Check sheet for the modelled part. Datum: model origin and axes. Units: mm. Face numbers are marked on the shaded views. A direction names the side the tool comes from. Round coordinates to 2 decimals unless told otherwise and drop trailing zeros. Order: outer loops, then holes, each group sorted by start corner. A loop starts at its lowest first (then second) coordinate and runs counter-clockwise, first axis right, second up.
Q1. Scan lines: probe 1 along Z at (x, y) = (177, -34.45); probe 2 along Y at (x, z) = (42, 2.75); probe 3 along Y at (x, z) = (145.5, 2). Record each from-to range of solid material in increasing order.
Q2. Cross-section at A-A on y = 1. Record the cut outline in (x, z).
Q3. Cross-section at C-C on y = -22. Record the cut outline in (x, z), then the cut area to 3 significant figures.
Q4. Set-up check for the marked faces 1, 2, 3 and 4: record each of +Z, -Z, +X, -X, +Y, -Y from which the full face is reachable in a straight line by a thin tool's end or side.
Q5. Cross-section at B-B on x = 84.5. Record the cut outline in (y, z).
Q6. Depth check by flat-ended pin: P1, Ø2, axis at x = 106, z = 2, coming from the -Y side; P2, Ø0.6, axis at x = 112, y = -38, coming from the -Z side; P3, Ø4, axis at x = 58.5, z = -21, coming from the +Y side; P4, Ø3, axis at x = 60, z = -6, coming from the -Y side. Enter the tip coordinate at first touch or a pass-through.
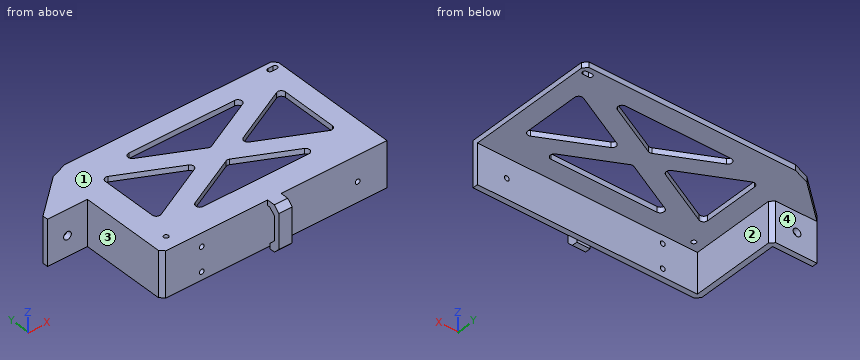
from build123d import *

# Parameters (mm, degrees)
SKETCH_R        = 1.75
PAD_DEPTH       = 4
PAD001_DEPTH    = 34
FILLET_R        = 3
CHAMFER_SIZE    = 3
SKETCH006_R     = 2.9
HOLE_DEPTH      = 25
HOLE_TIPS_R     = 2.9
SKETCH007_R     = 1.8
HOLE001_DEPTH   = 25
CHAMFER001_SIZE = 3
CHAMFER002_SIZE = 7
SKETCH008_W     = 10
SKETCH008_H     = 10
PAD002_DEPTH    = 4
SKETCH009_W     = 10
SKETCH009_H     = 4
PAD003_DEPTH    = 30
SKETCH010_W     = 10
SKETCH010_H     = 4
PAD004_DEPTH    = 4
CHAMFER003_SIZE = 3.99


with BuildPart() as part:
    # Sketch → Pad (new body)
    with BuildSketch(Plane.XY):
        Polygon((30, 0), (30, 30), (0, 30), (0, 34), (34, 64), (199, 64), (199, -33), (199, -37), (30, -37), (30, -33), align=None)
        with Locations((42, -26.5)):
            Circle(SKETCH_R, mode=Mode.SUBTRACT)
        Polygon((64, 49), (116.5, 23), (169, 49), align=None, mode=Mode.SUBTRACT)
        Polygon((116.5, 8), (64, -18), (169, -18), align=None, mode=Mode.SUBTRACT)
        Polygon((49, 41.5), (101.38806, 15.5), (49, -10.5), align=None, mode=Mode.SUBTRACT)
        Polygon((184, 41.5), (131.61194, 15.5), (184, -10.5), align=None, mode=Mode.SUBTRACT)
        with BuildLine():
            ThreePointArc((194.5, 56.75), (196.25, 58.5), (194.499999, 60.25))
            Line((194.5, 60.25), (190.5, 60.25))
            ThreePointArc((190.500001, 60.25), (188.75, 58.5), (190.5, 56.75))
            Line((194.5, 56.75), (190.5, 56.75))
        make_face(mode=Mode.SUBTRACT)
    extrude(amount=PAD_DEPTH)

    # Sketch001 (on Face24 of Pad) → Pad001 (join)
    with BuildSketch(Plane.XY.offset(4)):
        Polygon((30, 0), (30, 30), (0, 30), (0, 34), (34, 34), (34, -33), (199, -33), (199, -37), (30, -37), (30, -33), align=None)
    extrude(amount=-PAD001_DEPTH)

    # Fillet
    fillet_edges = [part.edges().sort_by_distance(p)[0] for p in [
        (49, 41.5, 2),
        (101.38806, 15.5, 2),
        (49, -10.5, 2),
        (64, -18, 2),
        (116.5, 8, 2),
        (169, -18, 2),
        (184, -10.5, 2),
        (64, 49, 2),
        (116.5, 23, 2),
        (131.61194, 15.5, 2),
        (184, 41.5, 2),
        (169, 49, 2),
    ]]
    fillet(fillet_edges, radius=FILLET_R)

    # Chamfer
    chamfer_edges = [part.edges().sort_by_distance(p)[0] for p in [
        (199, 64, 2),
    ]]
    chamfer(chamfer_edges, length=CHAMFER_SIZE)

    # Sketch006 (on Face6 of Chamfer) → Hole (cut)
    with BuildSketch(Plane(origin=(0, 34, 0), x_dir=(-1, 0, 0), z_dir=(0, 1, 0))):
        with Locations((-15, -15)):
            Circle(SKETCH006_R)
    extrude(amount=-HOLE_DEPTH, mode=Mode.SUBTRACT)

    # Hole tips → Hole tip 1 section 0
    with BuildSketch(Plane(origin=(0, 9, 0), x_dir=(-1, 0, 0), z_dir=(0, 1, 0)), mode=Mode.PRIVATE) as hole_tip_1_s0:
        with Locations((-15, -15)):
            Circle(HOLE_TIPS_R)
    loft([hole_tip_1_s0.sketch, Vertex(15, 7.257504, -15)], mode=Mode.SUBTRACT)

    # Sketch007 (on Face7 of Hole) → Hole001 (cut)
    with BuildSketch(Plane(origin=(0, -33, 0), x_dir=(-1, 0, 0), z_dir=(0, 1, 0))):
        with Locations((-177, -15)):
            Circle(SKETCH007_R)
        with Locations((-60, -6)):
            Circle(SKETCH007_R)
        with Locations((-60, -24)):
            Circle(SKETCH007_R)
    extrude(amount=-HOLE001_DEPTH, mode=Mode.SUBTRACT)

    # Chamfer001
    chamfer001_edges = [part.edges().sort_by_distance(p)[0] for p in [
        (30, -37, -13),
        (34, 34, -15),
    ]]
    chamfer(chamfer001_edges, length=CHAMFER001_SIZE)

    # Chamfer002
    chamfer002_edges = [part.edges().sort_by_distance(p)[0] for p in [
        (34, 64, 2),
    ]]
    chamfer(chamfer002_edges, length=CHAMFER002_SIZE)

    # Sketch008 (on Face41 of Chamfer002) → Pad002 (join)
    with BuildSketch(Plane.XY.offset(4)):
        with Locations((114.5, -42)):
            Rectangle(SKETCH008_W, SKETCH008_H)
    extrude(amount=-PAD002_DEPTH)

    # Sketch009 (on Face51 of Pad002) → Pad003 (join)
    with BuildSketch(Plane(origin=(0, 0, 0), x_dir=(1, 0, 0), z_dir=(0, 0, -1))):
        with Locations((114.5, 45)):
            Rectangle(SKETCH009_W, SKETCH009_H)
    extrude(amount=PAD003_DEPTH)

    # Sketch010 (on Face52 of Pad003) → Pad004 (join)
    with BuildSketch(Plane(origin=(0, -43, 0), x_dir=(-1, 0, 0), z_dir=(0, 1, 0))):
        with Locations((-114.5, -28)):
            Rectangle(SKETCH010_W, SKETCH010_H)
    extrude(amount=PAD004_DEPTH)

    # Chamfer003
    chamfer003_edges = [part.edges().sort_by_distance(p)[0] for p in [
        (114.5, -47, 4),
        (114.5, -47, -30),
        (114.5, -43, -26),
        (114.5, -43, 0),
    ]]
    chamfer(chamfer003_edges, length=CHAMFER003_SIZE)


solid = part.part
Results found:
1. probe 1: z = -30 to -16.8, -13.2 to 4
1. probe 2: y = -37 to -28.25, -24.75 to 64
1. probe 3: y = -37 to -18, -6.36 to 8.61, 22.39 to 37.36, 49 to 64
2. outline: (30, -30) - (34, -30) - (34, 0) - (49, 0) - (49, 4) - (30, 4) - close; (72.17, 0) - (102.37, 0) - (102.37, 4) - (72.17, 4) - close; (130.63, 0) - (160.83, 0) - (160.83, 4) - (130.63, 4) - close; (184, 0) - (199, 0) - (199, 4) - (184, 4) - close
3. outline: (30, -30) - (34, -30) - (34, 0) - (199, 0) - (199, 4) - (30, 4) - close
3. area: 796 mm2
4. face 1: +Z, +X, -X, +Y, -Y
4. face 2: -Z, +X, +Y
4. face 3: +Z, -Z, -X, -Y
4. face 4: -Z, +X, -X, +Y
5. outline: (-37, -30) - (-33, -30) - (-33, 0) - (-18, 0) - (-18, 4) - (-37, 4) - close; (-7.85, 0) - (7.12, 0) - (7.12, 4) - (-7.85, 4) - close; (23.88, 0) - (38.85, 0) - (38.85, 4) - (23.88, 4) - close; (49, 0) - (64, 0) - (64, 4) - (49, 4) - close
6. P1: stops at y = -37
6. P2: stops at z = 0
6. P3: stops at y = -33
6. P4: passes through
